from build123d import *

# Parameters (mm, degrees)
SKETCH1_W           = 25
SKETCH1_H           = 25
BOSS_EXTRUDE1_DEPTH = 5
SKETCH3_R           = 1.25
CUT_EXTRUDE1_DEPTH  = 19.371173071
SKETCH4_W           = 20
SKETCH4_H           = 20
CUT_EXTRUDE2_DEPTH  = 19.371173071
FILLET1_R           = 2.5


with BuildPart() as part:
    # Sketch1 → Boss-Extrude1 (new body)
    with BuildSketch(Plane(origin=(0, 0, 0), x_dir=(1, 0, 0), z_dir=(0, 1, 0))):
        Rectangle(SKETCH1_W, SKETCH1_H)
    extrude(amount=BOSS_EXTRUDE1_DEPTH)

    # Sketch3 → Cut-Extrude1 (cut, through all)
    with BuildSketch(Plane(origin=(0, 5, 0), x_dir=(1, 0, 0), z_dir=(0, 1, 0))):
        with Locations(Location((-10, 10, 0), (0, 0, 270))):
            Circle(SKETCH3_R)
        with Locations(Location((10, 10, 0), (0, 0, 270))):
            Circle(SKETCH3_R)
        with Locations(Location((-10, -10, 0), (0, 0, 270))):
            Circle(SKETCH3_R)
    extrude(amount=-CUT_EXTRUDE1_DEPTH, mode=Mode.SUBTRACT)

    # Sketch4 → Cut-Extrude2 (cut, through all)
    with BuildSketch(Plane(origin=(0, 5, 0), x_dir=(1, 0, 0), z_dir=(0, 1, 0))):
        with Locations((2.5, -2.5)):
            Rectangle(SKETCH4_W, SKETCH4_H)
    extrude(amount=-CUT_EXTRUDE2_DEPTH, mode=Mode.SUBTRACT)

    # Fillet1
    fillet1_edges = [part.edges().sort_by_distance(p)[0] for p in [
        (-12.5, 2.5, 12.5),
        (12.5, 2.5, -12.5),
        (-12.5, 2.5, -12.5),
        (12.5, 2.5, -7.5),
        (-7.5, 2.5, 12.5),
        (-7.5, 2.5, -7.5),
    ]]
    fillet(fillet1_edges, radius=FILLET1_R - 0.0001)  # a hair under: the kernel refuses the full size


solid = part.part
Work out the finished part from the listing and answer in its coordinate system (mm). A direction names the side the tool comes from. Give positions to 0.01 mm unless a question says otherwise; leave off trailing zeros. Loops run counter-clockwise (first coordinate to the right, second up) from the corner with the lowest first, then second, coordinate; pieces in that order, holes last. Notation, with made-up numbers: (42, 55.25) -> (65, 55.25) arc R9 cw to (65, 59.25) -> close; hole circle Ø9 at (-13, -18). An arc over 180 degrees is marked (long way). Use a Markdown table: item, result. Add a question column.
1. Section C-C on z = -2 is taken. Determine the outline of the cut face in (x, y), and give its area (3 significant figures).
2. Section B-B on x = 10.5 is taken. Determine the outline of the cut face in (y, z), and give its area (3 significant figures).
3. Section A-A on y = 0.65 is taken. State how many separate pieces and enclosed holes the cut face has, and give its area (3 significant figures).
4. Section D-D on x = 4.5 is taken. Determine the outline of the cut face in (y, z).
5. Determine the mould class of faces 1 (the flat face through (-7.5, 3, 3)), 2 (the cylindrical face through (-9.95, 2.54, 8.75)), 3 (the cylindrical face through (-8.252, 2.465, 11.787)) for opening direction Z: released by +Z, released by -Z, zero draft, split by the parting line, or undercut.
6. Find the intervals of material crossed by probe 1 along X at (y, z) = (1.1, -10); probe 2 along X at (y, z) = (3.1, 10); probe 3 along Z at (x, y) = (-1.25, 1.4), in increasing order.
7. Flat-ended cylindrical pins translate along their axes: pin 1 Ø1.5 at (y, z) = (1.5, 2.5) entering from +X; pin 2 Ø1.5 at (x, y) = (4, 1.5) entering from +Z; pin 3 Ø12 at (x, z) = (1.5, 1.5) entering from -Y. Find the tip coordinate at first contact, or state that the pin passes through.
8. For faces 4 (the flat face through (2, 3, -7.5)), 5 (the cylindrical face through (10.845, 2.535, -10.921)), determine the directions among +Z, -Z, +X, -X, +Y, -Y from which every point of the face is accessible in a straight line to the end or side of a thin tool.
Results below:
| question | item | result |
|---|---|---|
| 1 | outline | (-12.5, 0) -> (-7.5, 0) -> (-7.5, 5) -> (-12.5, 5) -> close |
| 1 | area | 25.0 mm^2 |
| 2 | outline | (0, -12.45) -> (5, -12.45) -> (5, -11.15) -> (0, -11.15) -> close; (0, -8.85) -> (5, -8.85) -> (5, -7.55) -> (0, -7.55) -> close |
| 2 | area | 13.0 mm^2 |
| 3 | separate pieces | 1 |
| 3 | enclosed holes | 3 |
| 3 | area | 205 mm^2 |
| 4 | outline | (0, -12.5) -> (5, -12.5) -> (5, -7.5) -> (0, -7.5) -> close |
| 5 | face 1 | zero draft |
| 5 | face 2 | undercut |
| 5 | face 3 | released by +Z |
| 6 | probe 1 | x = -12.5 to -11.25, -8.75 to 8.75, 11.25 to 12.5 |
| 6 | probe 2 | x = -12.5 to -11.25, -8.75 to -7.5 |
| 6 | probe 3 | z = -12.5 to -7.5 |
| 7 | pin 1 | stops at x = -7.5 |
| 7 | pin 2 | stops at z = -7.5 |
| 7 | pin 3 | passes through |
| 8 | face 4 | +Z, +X, +Y, -Y |
| 8 | face 5 | +Y, -Y |
